Geometry: see drawing. Coordinates: mm, zero at the bounding-box minimum. Coordinates: 2 decimals unless noted, no trailing zeros. Loops run counter-clockwise (first coordinate to the right, second up) from the corner with the lowest first, then second, coordinate; pieces in that order, holes last. Notation, with made-up numbers: (48, 7) -> (57, 7) arc R10 ccw to (57, 11) -> close; hole circle Ø6 at (-17.5, 29). An arc over 180 degrees is marked (long way). One line per question, with ' | ' between items. Start each with the question number.
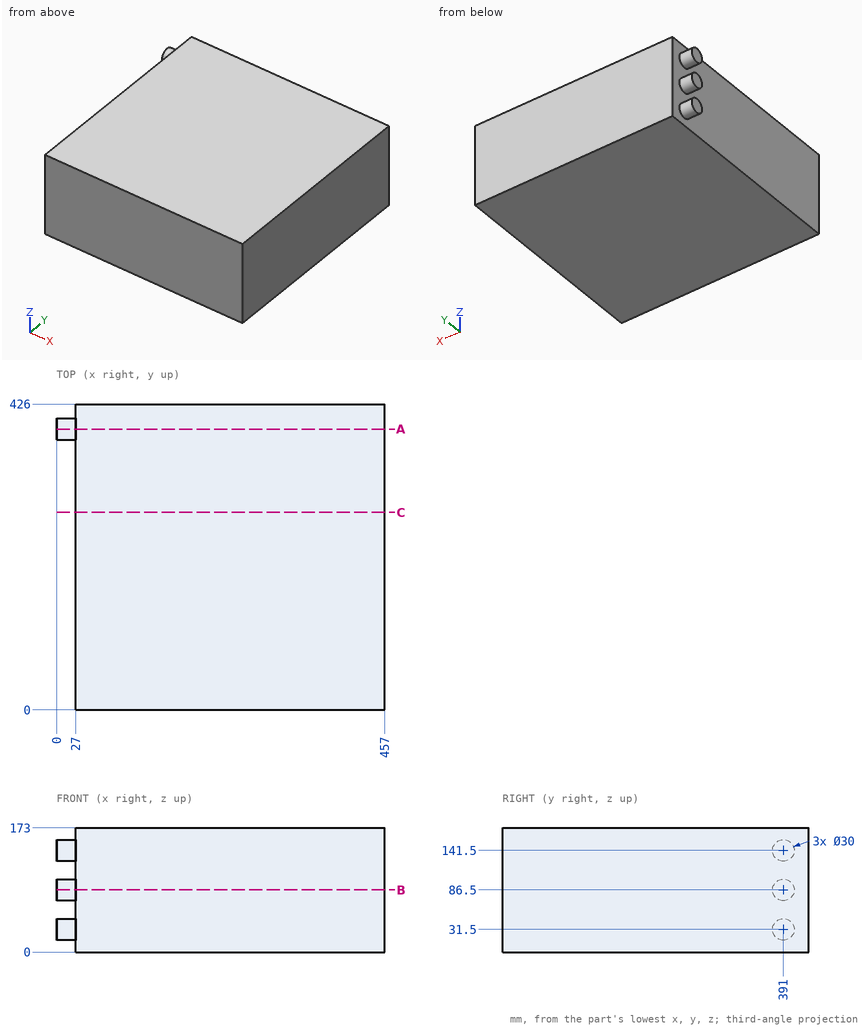
(1) Cut plane B-B, the plane z = 86.5. Return the cut outline in (x, y), and give its area (3 significant figures).
(2) Contact query for a flat-ended pin moving along its axis: pin 1 Ø6 at (y, z) = (112, 132.5) entering from -X. Output: stop coordinate, or through.
(3) Cut plane A-A, the plane y = 391. Return the cut outline in (x, z).
(4) Ray query, L1, parallel to X at y = 407, z = 37.5. Return the intervals inside material, ascending.
(5) Cut plane C-C, the plane y = 275. Return the cut outline in (x, z).
Here are the results:
1) outline: (0, 376) -> (27, 376) -> (27, 0) -> (457, 0) -> (457, 426) -> (27, 426) -> (27, 406) -> (0, 406) -> close | area: 184,000 mm2
2) pin 1: stops at x = 27
3) outline: (0, 16.5) -> (27, 16.5) -> (27, 0) -> (457, 0) -> (457, 173) -> (27, 173) -> (27, 156.5) -> (0, 156.5) -> (0, 126.5) -> (27, 126.5) -> (27, 101.5) -> (0, 101.5) -> (0, 71.5) -> (27, 71.5) -> (27, 46.5) -> (0, 46.5) -> close
4) L1: x = 27 to 457
5) outline: (27, 0) -> (457, 0) -> (457, 173) -> (27, 173) -> close
